Geometry check sheet. Reference: drawing and pictorial views, mm from the part's lowest x, y, z. Round coordinates to 2 decimals unless told otherwise and drop trailing zeros. Order: outer loops, then holes, each group sorted by start corner. A loop starts at its lowest first (then second) coordinate and runs counter-clockwise, first axis right, second up.
(1) Sectioned sample at B-B (z = 4.5). Record the boundary of the cut face in (x, y).
(2) Go/stop test with flat-tipped pins: pin 1 (3 mm diameter, centred on x = 81, y = 5, fed in from -Z); pin 2 (2 mm diameter, centred on x = 48.5, y = 65, fed in from +Z); pin 3 (5.5 mm diameter, centred on x = 59, z = 6.5, fed in from +Y). Record where each tip stops, or that it passes through.
(3) Release check for a two-part mould opening along Y. For the marked faces 1, 2, 3 and 4 record: +Y half, -Y half, draft (parallel to the pull), parting line (faces both ways), or undercut.
(4) Material ranges on line 1 along Y through (x, z) = (81, 3.25); line 2 along X through (y, z) = (96, 4.75); line 3 along X through (y, z) = (42, 9.25), recorded low to high.
(5) Sectioned sample at A-A (x = 36.5). Record the boundary of the cut face in (y, z).
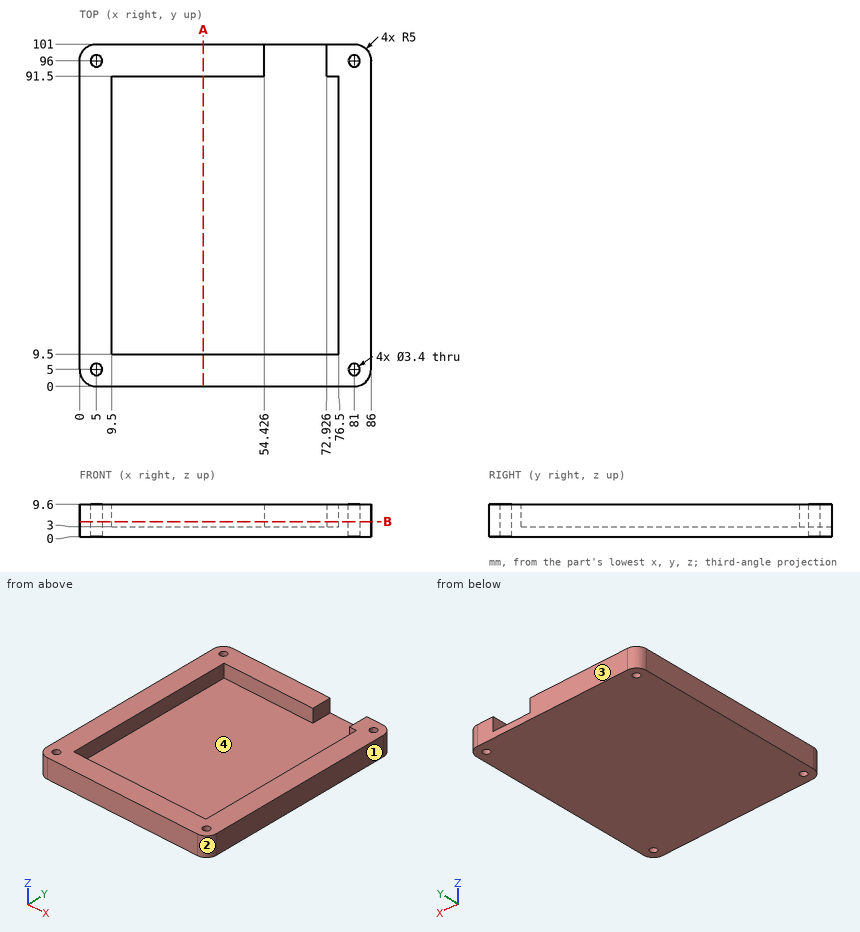
Answer below:
1. outline: (0, 5) arc R5 ccw to (5, 0) - (81, 0) arc R5 ccw to (86, 5) - (86, 96) arc R5 ccw to (81, 101) - (72.93, 101) - (72.93, 91.5) - (76.5, 91.5) - (76.5, 9.5) - (9.5, 9.5) - (9.5, 91.5) - (54.43, 91.5) - (54.43, 101) - (5, 101) arc R5 ccw to (0, 96) - close; hole circle Ø3.4 at (5, 5); hole circle Ø3.4 at (5, 96); hole circle Ø3.4 at (81, 5); hole circle Ø3.4 at (81, 96)
2. pin 1: passes through
2. pin 2: stops at z = 3
2. pin 3: stops at y = 9.5
3. face 1: draft
3. face 2: -Y half
3. face 3: +Y half
3. face 4: undercut
4. line 1: y = 0 to 3.3, 6.7 to 94.3, 97.7 to 101
4. line 2: x = 0 to 3.3, 6.7 to 54.43, 72.93 to 79.3, 82.7 to 86
4. line 3: x = 0 to 9.5, 76.5 to 86
5. outline: (0, 0) - (101, 0) - (101, 9.6) - (91.5, 9.6) - (91.5, 3) - (9.5, 3) - (9.5, 9.6) - (0, 9.6) - close
